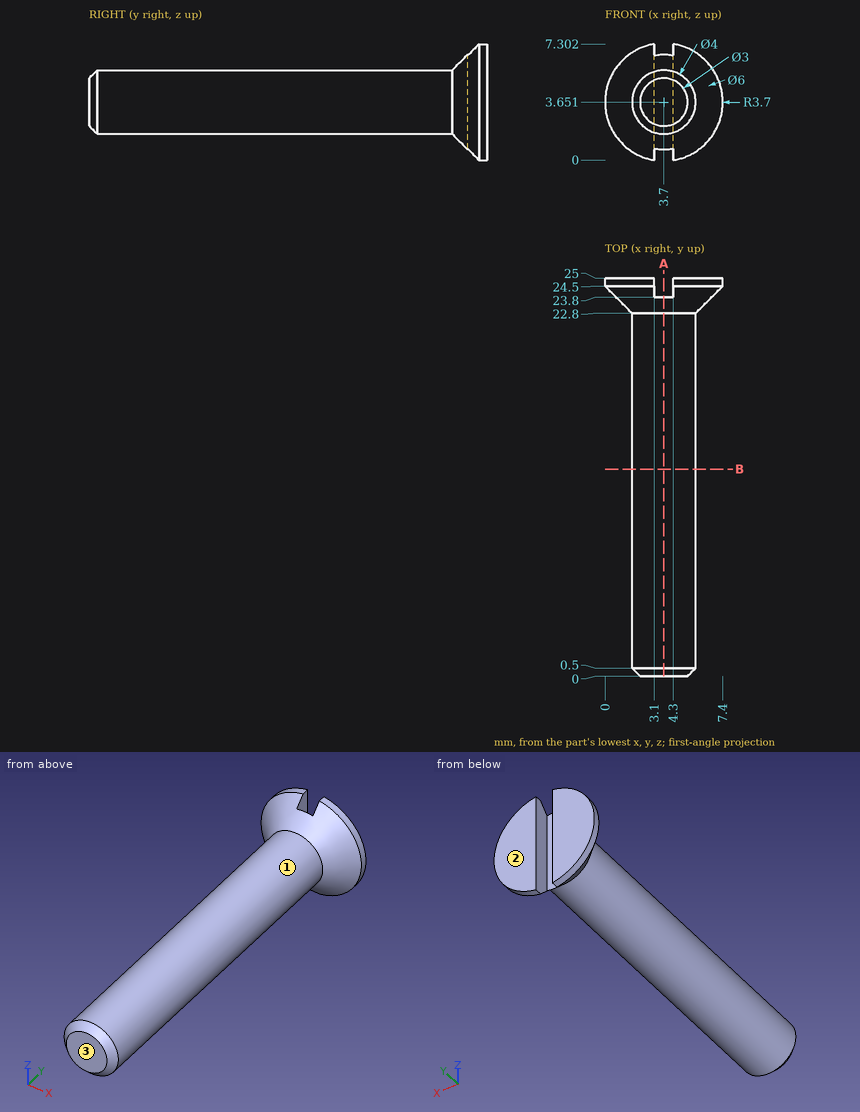
For this review, use the dimensioned drawing (mm, ordinates from the lowest corner) and the shaded views. Round coordinates to 2 decimals unless told otherwise and drop trailing zeros. Write each loop counter-clockwise with the first axis right and the second up, starting at its lowest first coordinate (ties: lowest second). Pieces come first, ordered by that corner, then holes. Notation, with made-up numbers: (36, 61) -> (42, 61) arc R26 ccw to (42, 84) -> close; hole circle Ø5 at (35.25, 85). An arc over 180 degrees is marked (long way). Answer in a Markdown table with one row per item.
Q1. Clearance check with flat-ended pins moving along their axes: pin 1 Ø3 at (y, z) = (7.5, 3.5) entering from -X; pin 2 Ø1.5 at (x, z) = (1.5, 4.5) entering from -Y; pin 3 Ø4 at (y, z) = (14.5, 4) entering from +X. State where each tip first meets the part, or that it passes through.
The answers:
| item | result |
|---|---|
| pin 1 | x = 1.7 |
| pin 2 | y = 0.11 |
| pin 3 | x = 5.7 |
Q2. Take a section at A-A, the plane x = 3.7. State the section outline as (y, z) points.
The answers:
| item | result |
|---|---|
| outline | (0, 2.15) -> (0.5, 1.65) -> (22.8, 1.65) -> (23.8, 0.65) -> (23.8, 6.65) -> (22.8, 5.65) -> (0.5, 5.65) -> (0, 5.15) -> close |
Q3. Draft analysis for pull direction Y (two halves, no side actions). For the marked faces 1, 2 and 3, state which applies: +Y half, -Y half, draft (parallel to the pull), parting line (faces both ways), or undercut.
The answers:
| item | result |
|---|---|
| face 1 | draft |
| face 2 | +Y half |
| face 3 | -Y half |
Q4. Take a section at B-B, the plane y = 13. State the section outline as (x, z) points, then the cut area to 3 significant figures.
The answers:
| item | result |
|---|---|
| outline | circle Ø4 at (3.7, 3.65) |
| area | 12.6 mm² |
Q5. To check wall thickness, follow L1, parallel to Y at x = 3.75, z = 4.75; L2, parallel to X at y = 20.25, z = 3.5; L3, parallel to Y at x = 6.5, z = 4. State the ranges of each line that lie inside material, in increasing order. Write a range as [from, to].
The answers:
| item | result |
|---|---|
| L1 | [0, 23.8] |
| L2 | [1.71, 5.69] |
| L3 | [23.62, 25] |
